For this review, take the finished solid that the model builds, in its own axes (mm). A direction names the side the tool comes from. Coordinates: 2 decimals unless noted, no trailing zeros. Write each loop counter-clockwise with the first axis right and the second up, starting at its lowest first coordinate (ties: lowest second). Pieces come first, ordered by that corner, then holes. Notation, with made-up numbers: (26, 0) -> (83, 0) arc R17 cw to (83, 5) -> close; hole circle Ø9 at (1.25, 60.25). An arc over 180 degrees is marked (long way). One line per item, written item: value. Start each with the question number.
1) Machinability: for faces 1 (the cylindrical face through (33.98, 105.28, 76.02)), 2 (the flat face through (31, 25.4, 34)), 3 (the flat face through (63.5, 65, 29)), which of the approach directions +Z, -Z, +X, -X, +Y, -Y give a long, thin tool a straight path to every point of the face, cutting with its end or side? Answer none if there is none.
2) Add section B-B (x = 6). State the section outline as (y, z) points, and give its area (3 significant figures).
3) Add section A-A (z = 51). State the section outline as (x, y) points.
4) For probe 1 along X at (y, z) = (51, 56); probe 2 along Z at (x, y) = (31.5, 23.5); probe 3 along Y at (x, z) = (31, 55.5), list the stretches that pass through material, from the lowest coordinate up. Write a range as from..to.
5) Mouldability with a two-part tool opening along X and no side actions: class faces 4 (the cylindrical face through (29.619, 1.528, 62.051)), 5 (the flat face through (27, 33.531, 51)), 6 (the flat face through (0, 63, 31)) as released by +X, released by -X, zero draft, split by the parting line, or undercut.
6) Add section C-C (y = 72). State the section outline as (x, z) points, and give its area (3 significant figures).
7) For pin 1 Ø20.5 at (y, z) = (42.5, 52.5) entering from -X; pin 2 Ø10 at (x, z) = (30.5, 65) entering from -Y; pin 3 Ø1 at (x, y) = (42, 71) entering from +Z; pin 4 Ø8 at (x, y) = (29.5, 43) entering from +Z, all flat-tipped, find the tip position at first contact; note any pin that passes through.
8) Add section D-D (z = 41.5). State the section outline as (x, y) points.
from build123d import *

# Parameters (mm, degrees)
F0_W     = 63.5
F0_H     = 63.5
F1_DEPTH = 127
F2_R     = 5.08
F3_SIZE  = 5.08
F4_W     = 29.269816
F4_H     = 26.25883
F5_DEPTH = 25.4
F4_R     = 13.374611
F6_DEPTH = 25.4
F7_R     = 14.75744
F8_DEPTH = 25.4


with BuildPart() as f1:
    # F0 (on Front) → F1 (new body)
    with BuildSketch(Plane.XZ):
        with Locations((31.75, 31.75)):
            Rectangle(F0_W, F0_H)
    extrude(amount=-F1_DEPTH)

    # F2
    f2_edges = [f1.edges().sort_by_distance(p)[0] for p in [
        (31.75, 0, 63.5),
    ]]
    fillet(f2_edges, radius=F2_R)

    # F3
    f3_edges = [f1.edges().sort_by_distance(p)[0] for p in [
        (63.5, 66.04, 63.5),
        (63.5, 0, 29.21),
    ]]
    chamfer(f3_edges, length=F3_SIZE)

    # F4 (on face) → F5 (cut)
    with BuildSketch(Plane.XY.offset(63.5)):
        with Locations((26.733129, 46.660667)):
            Rectangle(F4_W, F4_H)
    extrude(amount=-F5_DEPTH, mode=Mode.SUBTRACT)

    # F4 (on face) → F6 (join)
    with BuildSketch(Plane.XY.offset(63.5)):
        with Locations((26.789799, 94.000928)):
            Circle(F4_R)
    extrude(amount=F6_DEPTH)

    # F7 (on face) → F8 (cut)
    with BuildSketch(Plane.XZ):
        with Locations((31.600073, 33.965837)):
            Circle(F7_R)
    extrude(amount=-F8_DEPTH, mode=Mode.SUBTRACT)


solid = f1.part
Numbers:
1. face 1: +Z
1. face 2: -Y
1. face 3: +Z, -Z, +X, +Y, -Y
2. outline: (0, 0) -> (127, 0) -> (127, 63.5) -> (5.08, 63.5) arc R5.08 ccw to (0, 58.42) -> close
2. area: 8,060 mm²
3. outline: (0, 0) -> (58.42, 0) -> (63.5, 5.08) -> (63.5, 127) -> (0, 127) -> close; hole (12.1, 33.53) -> (41.37, 33.53) -> (41.37, 59.79) -> (12.1, 59.79) -> close
4. probe 1: 0..12.1, 41.37..63.5
4. probe 2: 0..19.21, 48.72..63.5
4. probe 3: 0..33.53, 59.79..127
5. face 4: zero draft
5. face 5: undercut
5. face 6: released by -X
6. outline: (0, 0) -> (63.5, 0) -> (63.5, 58.42) -> (58.42, 63.5) -> (0, 63.5) -> close
6. area: 4,020 mm²
7. pin 1: x = 0
7. pin 2: y = 0.25
7. pin 3: z = 63.5
7. pin 4: z = 38.1
8. outline: (0, 0) -> (18.91, 0) -> (18.91, 25.4) -> (44.29, 25.4) -> (44.29, 0) -> (58.42, 0) -> (63.5, 5.08) -> (63.5, 127) -> (0, 127) -> close; hole (12.1, 33.53) -> (41.37, 33.53) -> (41.37, 59.79) -> (12.1, 59.79) -> close
